Study the drawing (mm; zero at the part's minimum x, y, z) and answer. A direction names the side the tool comes from. Coordinates: 2 decimals unless noted, no trailing zeros. Order: outer loops, then holes, each group sorted by start corner. A loop starts at its lowest first (then second) coordinate and runs counter-clockwise, first axis right, second up. Notation, with made-up numbers: M -5,72.25 L 52,72.25 A22 cw 52,87.25 Z; hole C -39,55.5 d9. An arc over 180 degrees is marked long. One line per item, written item: value. Start each with the question number.
Q1. The part is cut by section A-A on z = 2.75. Give the vertices of the cut face in (x, y), then the cut area to 3 significant figures.
Q2. The part is cut by section B-B on y = 30. Give the vertices of the cut face in (x, z).
Q3. For the marked faces 1, 2 and 3, determine the directions among +Z, -Z, +X, -X, +Y, -Y from which every point of the face is accessible in a straight line to the end or side of a thin tool.
Q4. The part is cut by section D-D on z = 17.75. Give the vertices of the cut face in (x, y).
Q5. The part is cut by section C-C on x = 21.75. Give the vertices of the cut face in (y, z), then the cut area to 3 significant figures.
Q6. Determine the mould class of the marked faces 4, 5 and 6 for opening direction X: pulls with the +X half, pulls with the -X half, needs draft (parallel to the pull), parting line crosses it, or undercut.
Q7. Each of these flat-tipped pins is pushed along its axis until it touches: pin 1 Ø1 at (y, z) = (17, 18.5) entering from -X; pin 2 Ø2 at (x, z) = (20, 4) entering from +Y; pin 3 Ø3 at (y, z) = (6.5, 2.5) entering from -X; pin 4 Ø1.6 at (y, z) = (37, 18.5) entering from +X. Where does it stop, or does it pass through?
Q8. Straight lines are drawn through the part: line 1 along X through (y, z) = (34.5, 4.75); line 2 along Y through (x, z) = (21.5, 5.75); line 3 along X through (y, z) = (38, 2.5). For each, find the intervals that lie inside material, in ascending order. Write a range as [from, to].
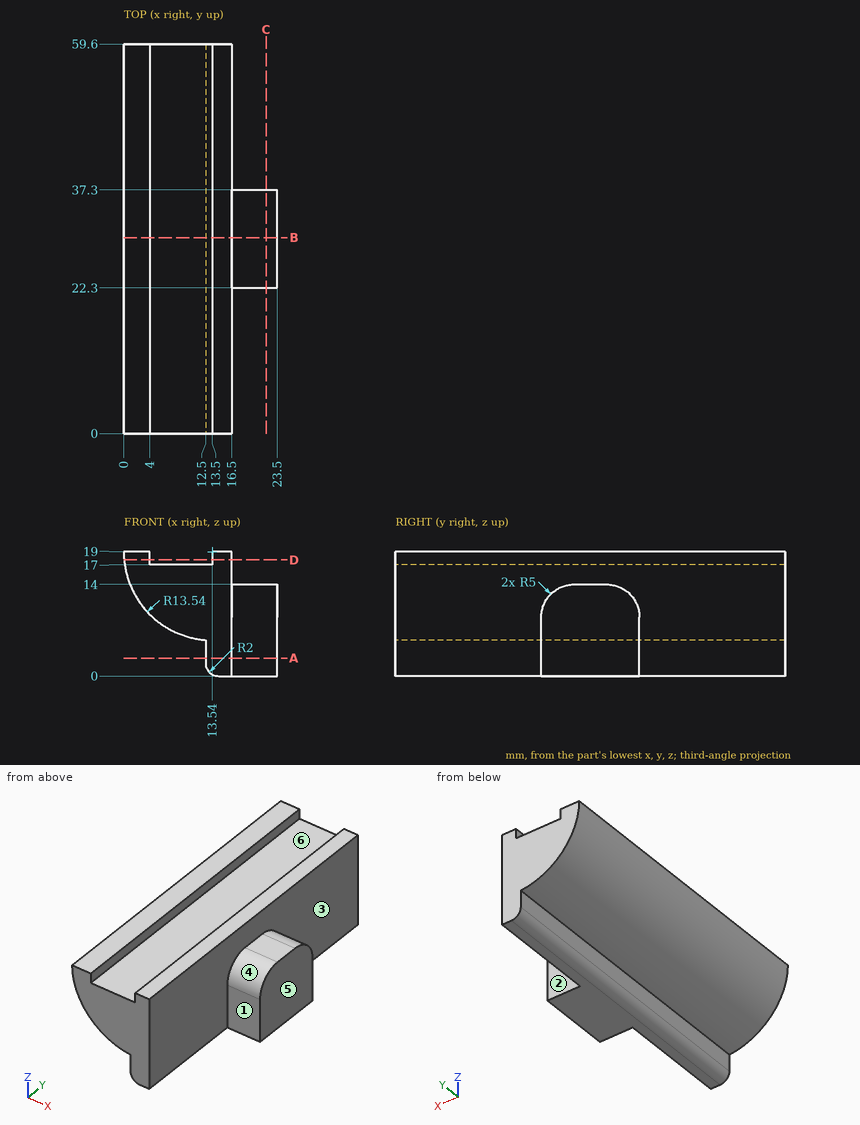
Output:
1. outline: M 12.5,0 L 16.5,0 L 16.5,22.3 L 23.5,22.3 L 23.5,37.3 L 16.5,37.3 L 16.5,59.6 L 12.5,59.6 Z
1. area: 343 mm^2
2. outline: M 0,19 A13.54 ccw 12.5,5.5 L 12.5,2 A2 ccw 14.5,0 L 23.5,0 L 23.5,14 L 16.5,14 L 16.5,19 L 13.5,19 L 13.5,17 L 4,17 L 4,19 Z
3. face 1: +Z, -Z, +X, -Y
3. face 2: +Z, -Z, +X, +Y
3. face 3: +Z, +X
4. outline: M 0.06,0 L 4,0 L 4,59.6 L 0.06,59.6 Z; M 13.5,0 L 16.5,0 L 16.5,59.6 L 13.5,59.6 Z
5. outline: M 22.3,0 L 37.3,0 L 37.3,9 A5 ccw 32.3,14 L 27.3,14 A5 ccw 22.3,9 Z
5. area: 199 mm^2
6. face 4: needs draft
6. face 5: pulls with the +X half
6. face 6: undercut
7. pin 1: stops at x = 0
7. pin 2: stops at y = 37.3
7. pin 3: stops at x = 12.5
7. pin 4: stops at x = 16.5
8. line 1: x = [12.5, 23.5]
8. line 2: y = [22.3, 37.3]
8. line 3: x = [12.5, 16.5]
